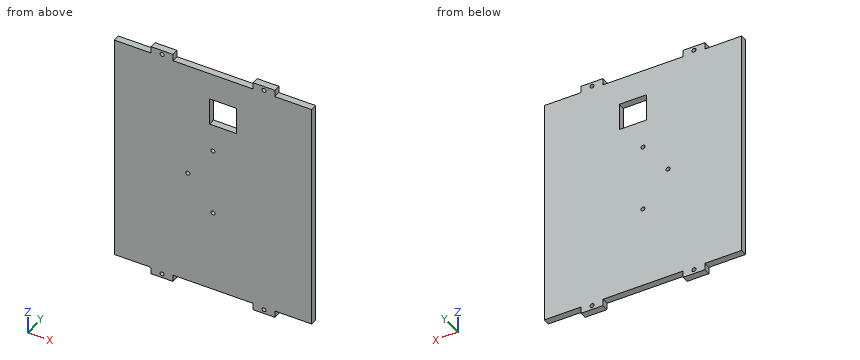
```python
from build123d import *

# Parameters (mm, degrees)
CROQUIS1_W                = 145.14
CROQUIS1_H                = 180
SALIENTE_EXTRUIR1_DEPTH   = 5
CROQUIS2_W                = 59
CROQUIS2_H                = 5
CROQUIS2_W_2              = 27.07
CORTAR_EXTRUIR1_DEPTH     = 116.721237895
CROQUIS3_R                = 1.5
CORTAR_EXTRUIR2_DEPTH     = 116.721237895
SIMETR_A3_COPY_1_SKETCH_R = 1.5
SIMETR_A3_COPY_1_DEPTH    = 116.721237895
CROQUIS4_R                = 1.5
CORTAR_EXTRUIR3_DEPTH     = 116.721237895
CROQUIS5_W                = 20
CROQUIS5_H                = 20
CORTAR_EXTRUIR4_DEPTH     = 116.721237895


with BuildPart() as part:
    # Croquis1 → Saliente-Extruir1 (new body)
    with BuildSketch(Plane(origin=(0, 0, 0), x_dir=(1, 0, 0), z_dir=(0, 1, 0))):
        Rectangle(CROQUIS1_W, CROQUIS1_H)
    extrude(amount=SALIENTE_EXTRUIR1_DEPTH)

    # Croquis2 → Cortar-Extruir1 (cut, through all)
    with BuildSketch(Plane(origin=(0, 5, 0), x_dir=(1, 0, 0), z_dir=(0, 1, 0))):
        with Locations((0, 87.5)):
            Rectangle(CROQUIS2_W, CROQUIS2_H)
        with Locations((-59.035, 87.5)):
            Rectangle(CROQUIS2_W_2, CROQUIS2_H)
        with Locations((59.035, 87.5)):
            Rectangle(CROQUIS2_W_2, CROQUIS2_H)
    cortar_extruir1 = extrude(amount=-CORTAR_EXTRUIR1_DEPTH, mode=Mode.SUBTRACT)

    # Simetría1: Cortar-Extruir1 across plane
    add(cortar_extruir1.mirror(Plane.XY), mode=Mode.SUBTRACT)

    # Croquis3 → Cortar-Extruir2 (cut, through all)
    with BuildSketch(Plane(origin=(0, 5, 0), x_dir=(1, 0, 0), z_dir=(0, 1, 0))):
        with Locations(Location((-37.5, 87, 0), (0, 0, 270))):
            Circle(CROQUIS3_R)
    cortar_extruir2 = extrude(amount=-CORTAR_EXTRUIR2_DEPTH, mode=Mode.SUBTRACT)

    # Simetría2: Cortar-Extruir2 across plane
    add(cortar_extruir2.mirror(Plane(origin=(0, 0, 0), x_dir=(0, 0, 1), z_dir=(1, 0, 0))), mode=Mode.SUBTRACT)

    # Simetría3: Cortar-Extruir2 across plane
    add(cortar_extruir2.mirror(Plane.XY), mode=Mode.SUBTRACT)

    # Simetría3 copy 1 sketch → Simetría3 copy 1 (cut, through all)
    with BuildSketch(Plane(origin=(0, 5, 0), x_dir=(-1, 0, 0), z_dir=(0, 1, 0))):
        with Locations(Location((-37.5, 87, 0), (0, 0, 270))):
            Circle(SIMETR_A3_COPY_1_SKETCH_R)
    extrude(amount=-SIMETR_A3_COPY_1_DEPTH, mode=Mode.SUBTRACT)

    # Croquis4 → Cortar-Extruir3 (cut, through all)
    with BuildSketch(Plane(origin=(0, 5, 0), x_dir=(1, 0, 0), z_dir=(0, 1, 0))):
        with Locations(Location((0, 24.5, 0), (0, 0, 270))):
            Circle(CROQUIS4_R)
        with Locations(Location((0, -24.5, 0), (0, 0, 270))):
            Circle(CROQUIS4_R)
        with Locations(Location((-18.5, 0, 0), (0, 0, 270))):
            Circle(CROQUIS4_R)
    extrude(amount=-CORTAR_EXTRUIR3_DEPTH, mode=Mode.SUBTRACT)

    # Croquis5 → Cortar-Extruir4 (cut, through all)
    with BuildSketch(Plane(origin=(0, 5, 0), x_dir=(1, 0, 0), z_dir=(0, 1, 0))):
        with Locations((7.43, -55)):
            Rectangle(CROQUIS5_W, CROQUIS5_H)
    extrude(amount=-CORTAR_EXTRUIR4_DEPTH, mode=Mode.SUBTRACT)


solid = part.part
```
For this review, take the finished solid that the model builds, in its own axes (mm). Round coordinates to 2 decimals unless told otherwise and drop trailing zeros. Write each loop counter-clockwise with the first axis right and the second up, starting at its lowest first coordinate (ties: lowest second). Pieces come first, ordered by that corner, then holes. Notation, with made-up numbers: (37.5, 56.25) -> (90.5, 56.25) arc R25 ccw to (90.5, 87.25) -> close; hole circle Ø9 at (-4, -19.75). An arc over 180 degrees is marked (long way). One line per question, with ' | ' between items. Start each with the question number.
1) For pin 1 Ø2.5 at (x, y) = (-5.5, 2.5) entering from +Z; pin 2 Ø1.5 at (x, y) = (7.5, 2) entering from -Z; pin 3 Ø1.5 at (y, z) = (1.5, -88) entering from -X, all flat-tipped, find the tip position at first contact; note any pin that passes through.
2) Add section A-A (y = 0.75). Count the separate pieces of the cut face and the enclosed holes in it, and give its area (3 significant figures).
3) Add section C-C (x = 64). Write out the cut boundary in (y, z), and give its area (3 significant figures).
4) Add section B-B (z = 61). Write out the cut boundary in (x, y).
5) Wall thickness on line 1 along X through (y, z) = (1.8, -87); line 2 along Z through (x, y) = (37.5, 3.3); line 3 along Z through (x, y) = (-2, 2): over which ranges is each line inside the solid? List them lowest first.
Reported:
1) pin 1: stops at z = 85 | pin 2: stops at z = -85 | pin 3: stops at x = -45.5
2) separate pieces: 1 | enclosed holes: 8 | area: 24,500 mm²
3) outline: (0, -85) -> (5, -85) -> (5, 85) -> (0, 85) -> close | area: 850 mm²
4) outline: (-72.57, 0) -> (-2.57, 0) -> (-2.57, 5) -> (-72.57, 5) -> close; (17.43, 0) -> (72.57, 0) -> (72.57, 5) -> (17.43, 5) -> close
5) line 1: x = -45.5 to -39, -36 to -29.5, 29.5 to 36, 39 to 45.5 | line 2: z = -90 to -88.5, -85.5 to 85.5, 88.5 to 90 | line 3: z = -85 to 45, 65 to 85
